The model under review builds one solid part; all positions refer to its coordinate system, in mm. Give positions to 0.01 mm unless a question says otherwise; leave off trailing zeros. Order: outer loops, then holes, each group sorted by start corner. A loop starts at its lowest first (then second) coordinate and runs counter-clockwise, first axis right, second up. Notation, with made-up numbers: M 62,-15 L 67,-15 A18 cw 67,-7 Z; hole C -14,40 d1. An arc over 180 degrees is marked long. One line per question, with ' | ' between items. Start each with the question number.
1. Wall thickness on L1, parallel to Y at x = 8.5, z = 0.6; L2, parallel to X at y = -22.5, z = 1.05; L3, parallel to Y at x = -1, z = 1.4: over which ranges is each line inside the solid? List them lowest first.
2. We need section C-C on y = -3. Write out the cut boundary in (x, z), then the cut area to 3 significant figures.
3. We need section D-D on x = -3.5. Write out the cut boundary in (y, z), then the cut area to 3 significant figures.
4. We need section A-A on z = 1.2. Write out the cut boundary in (x, y).
5. We need section B-B on x = 9.5. Write out the cut boundary in (y, z).
6. Insertion check: P1, Ø1.5, axis at y = -10, z = 0.5, coming from the +X side; P2, Ø0.8, axis at x = 14.5, z = 1.5, coming from the +Y side; P3, Ø5, axis at x = -43, y = -21.5, coming from the -Z side; P4, Ø0.8, axis at x = 13.5, z = 1.5, coming from the -Y side. Each pin has a flat end and moves straight along its axis. Give the tip position at first contact, or say it passes through.
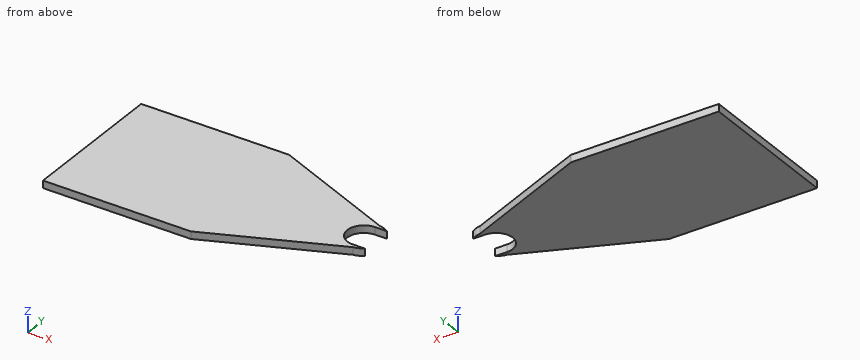
```python
from build123d import *

# Parameters (mm, degrees)
F0_W     = 54
F0_H     = 54
F1_DEPTH = 2.7


# Not quite as in the source:
# - a feature names something its author has since deleted; it is built from what else it names


with BuildPart() as f1:
    # F0 (on Top) → F1 (new body)
    with BuildSketch(Plane.XY):
        with Locations((-60.3654519308, -7.9408198703)):
            Rectangle(F0_W, F0_H)
        with BuildLine():
            Line((-33.3654519308, -34.9408198703), (12.8123124507, -15.3844278592))
            ThreePointArc((12.8123124507, -15.3844278592), (14.6191753291, -14.9283225153), (16.2578103101, -14.0408198703))
            Line((16.2578103101, -14.0408198703), (11.8943254642, -14.0408198703))
            ThreePointArc((11.8943254642, -14.0408198703), (5.7943254642, -7.9408198703), (11.8943254642, -1.8408198703))
            Line((11.8943254642, -1.8408198703), (16.2578103101, -1.8408198703))
            ThreePointArc((16.2578103101, -1.8408198703), (14.6191753291, -0.9533172253), (12.8123124507, -0.4972118814))
            Line((12.8123124507, -0.4972118814), (-33.3654519308, 19.0591801297))
            Line((-33.3654519308, 19.0591801297), (-33.3654519308, -34.9408198703))
        make_face()
    extrude(amount=F1_DEPTH)


solid = f1.part
```
Entries:
1) L1: y = -17.21 to -13.01, -2.87 to 1.33 | L2: x = -87.37 to -3.99 | L3: y = -21.23 to 5.35
2) outline: M -87.37,0 L 8.32,0 L 8.32,2.7 L -87.37,2.7 Z | area: 258 mm^2
3) outline: M -22.29,0 L 6.41,0 L 6.41,2.7 L -22.29,2.7 Z | area: 77.5 mm^2
4) outline: M -87.37,-34.94 L -33.37,-34.94 L 12.81,-15.38 A7.5 ccw 16.26,-14.04 L 11.89,-14.04 A6.1 cw 11.89,-1.84 L 16.26,-1.84 A7.5 ccw 12.81,-0.5 L -33.37,19.06 L -87.37,19.06 Z
5) outline: M -16.79,0 L -13.55,0 L -13.55,2.7 L -16.79,2.7 Z; M -2.33,0 L 0.91,0 L 0.91,2.7 L -2.33,2.7 Z
6) P1: stops at x = 6.48 | P2: stops at y = -0.77 | P3: stops at z = 0 | P4: stops at y = -15.34
